from build123d import *

# Parameters (mm, degrees)
F0_R     = 57.5
F0_R_2   = 55.5
F1_DEPTH = 25
F2_R     = 57.5
F2_R_2   = 55.5
F2_R_3   = 50.75
F3_DEPTH = 3
F2_R_4   = 71.25
F4_DEPTH = 3
F5_R     = 71.25
F5_R_2   = 68.75
F6_DEPTH = 45


with BuildPart() as f1:
    # F0 (on Top) → F1 (new body)
    with BuildSketch(Plane.XY):
        Circle(F0_R)
        Circle(F0_R_2, mode=Mode.SUBTRACT)
    extrude(amount=F1_DEPTH)

    # F2 (on face) → F3 (join)
    with BuildSketch(Plane.XY.offset(25)):
        Circle(F2_R)
        Circle(F2_R_2, mode=Mode.SUBTRACT)
        Circle(F2_R_2)
        with Locations((0.2079256644, 0.1388053244)):
            Circle(F2_R_3, mode=Mode.SUBTRACT)
    extrude(amount=F3_DEPTH)

    # F2 (on face) → F4 (join)
    with BuildSketch(Plane.XY.offset(25)):
        Circle(F2_R_4)
        Circle(F2_R, mode=Mode.SUBTRACT)
    extrude(amount=F4_DEPTH)

    # F5 (on face) → F6 (join)
    with BuildSketch(Plane.XY.offset(28)):
        Circle(F5_R)
        Circle(F5_R_2, mode=Mode.SUBTRACT)
    extrude(amount=F6_DEPTH)


solid = f1.part
Can you work these out from the model? Positions are in its coordinate system, mm. A direction names the side the tool comes from. Give positions to 0.01 mm unless a question says otherwise; leave off trailing zeros. Order: outer loops, then holes, each group sorted by start corner. A loop starts at its lowest first (then second) coordinate and runs counter-clockwise, first axis right, second up. Notation, with made-up numbers: (32.5, 6.25) - (76.5, 6.25) arc R9 cw to (76.5, 21.25) - close; hole circle Ø6 at (-14.75, -1). An arc over 180 degrees is marked (long way). Write each question's results on one line, items separated by ' | '.
1) If we mould it in two halves opening along Y, with no side actions, what happens to faces 4 (the face through (-48, 32, 25)), 5 (the face through (-12.465, -56.133, 12.325)), 6 (the face through (-10.794, -49.404, 26.479))? For each: pulls with the +Y half, pulls with the -Y half, needs draft (parallel to the pull), parting line crosses it, or undercut.
Final values:
face 4: needs draft | face 5: parting line crosses it | face 6: undercut
2) Please list where these lines run through material, in increasing order: line 1 along Y through (x, z) = (0, 53.5); line 2 along Y through (x, z) = (0, 17); line 3 along Z through (x, y) = (-46, -50.5). Write a range as [from, to].
Final values:
line 1: y = [-71.25, -68.75], [68.75, 71.25] | line 2: y = [-57.5, -55.5], [55.5, 57.5] | line 3: z = [25, 28]
3) On a 3-axis mill with a long thin cutter (end or side, diameter ignored), from which of +Z, -Z, +X, -X, +Y, -Y can I reach the whole of each face in a straight line? I mean faces 1 (the face through (24, -45, 25)), 2 (the face through (-52.514, 48.154, 48.664)), 3 (the face through (65.575, 20.651, 50.185)). Say none if no direction works.
Final values:
face 1: -Z | face 2: +Z, -Z | face 3: +Z
4) Suppose I cut it at B-B, the plane x = 46. Write out the boundary of the cut face in (y, z).
Final values:
outline: (-54.41, 25) - (-34.5, 25) - (-34.5, 0) - (-31.05, 0) - (-31.05, 25) - (-21.74, 25) - (-21.74, 28) - (-51.09, 28) - (-51.09, 73) - (-54.41, 73) - close; (22.02, 25) - (31.05, 25) - (31.05, 0) - (34.5, 0) - (34.5, 25) - (54.41, 25) - (54.41, 73) - (51.09, 73) - (51.09, 28) - (22.02, 28) - close
5) Suppose I cut it at C-C, the plane z = 7. Write out the boundary of the cut face in (x, y), then the cut area to 3 significant figures.
Final values:
outline: circle Ø115 at (0, 0); hole circle Ø111 at (0, 0) | area: 710 mm^2
6) Suppose I cut it at A-A, the plane y = 4.5. Write out the boundary of the cut face in (x, z), then the cut area to 3 significant figures.
Final values:
outline: (-71.11, 25) - (-57.32, 25) - (-57.32, 0) - (-55.32, 0) - (-55.32, 25) - (-50.35, 25) - (-50.35, 28) - (-68.6, 28) - (-68.6, 73) - (-71.11, 73) - close; (50.77, 25) - (55.32, 25) - (55.32, 0) - (57.32, 0) - (57.32, 25) - (71.11, 25) - (71.11, 73) - (68.6, 73) - (68.6, 28) - (50.77, 28) - close | area: 449 mm^2
7) Suppose I cut it at D-D, the plane z = 34. Write out the boundary of the cut face in (x, y), then the cut area to 3 significant figures.
Final values:
outline: circle Ø142.5 at (0, 0); hole circle Ø137.5 at (0, 0) | area: 1,100 mm^2
8) I'm going to push flat-ended pins straight in: pin 1 Ø5 at (y, z) = (19.5, 31.5) entering from +X; pin 2 Ø12 at (y, z) = (-20, 62.5) entering from -X; pin 3 Ø12 at (y, z) = (-35, 24) entering from -X. Where does each tip first touch, or does it pass through?
Final values:
pin 1: stops at x = 69.19 | pin 2: stops at x = -69.86 | pin 3: stops at x = -65.04
